from build123d import *

# Parameters (mm, degrees)
SKETCH_1_R          = 13.5
SKETCH_1_R_2        = 10
EXTRUDE_1_DEPTH     = 4
SKETCH_2_R          = 12.5
SKETCH_2_R_2        = 12.2
SKETCH_2_R_3        = 11.3
SKETCH_2_R_4        = 11
CUT_EXTRUDE_1_DEPTH = 0.3


with BuildPart() as part:
    # 草图1 → 凸台-拉伸1 (new body)
    with BuildSketch(Plane(origin=(0, 0, 0), x_dir=(1, 0, 0), z_dir=(0, 1, 0))):
        with Locations(Location((0, 0, 0), (0, 0, 270))):
            Circle(SKETCH_1_R)
        with Locations(Location((0, 0, 0), (0, 0, 270))):
            Circle(SKETCH_1_R_2, mode=Mode.SUBTRACT)
    extrude(amount=EXTRUDE_1_DEPTH)

    # 草图2 → 切除-拉伸1 (cut)
    # profile 1 of 2: a face of its own
    with BuildSketch(Plane(origin=(0, 4, 0), x_dir=(1, 0, 0), z_dir=(0, 1, 0))):
        with Locations(Location((0, 0, 0), (0, 0, 270))):
            Circle(SKETCH_2_R)
        with Locations(Location((0, 0, 0), (0, 0, 270))):
            Circle(SKETCH_2_R_2, mode=Mode.SUBTRACT)
    # profile 2 of 2: a face of its own
    with BuildSketch(Plane(origin=(0, 4, 0), x_dir=(1, 0, 0), z_dir=(0, 1, 0))):
        with Locations(Location((0, 0, 0), (0, 0, 270))):
            Circle(SKETCH_2_R_3)
        with Locations(Location((0, 0, 0), (0, 0, 270))):
            Circle(SKETCH_2_R_4, mode=Mode.SUBTRACT)
    cut_extrude_1 = extrude(amount=-CUT_EXTRUDE_1_DEPTH, mode=Mode.SUBTRACT)

    # 镜向1: 切除-拉伸1 across plane
    add(cut_extrude_1.mirror(Plane.ZX.offset(2)), mode=Mode.SUBTRACT)


solid = part.part
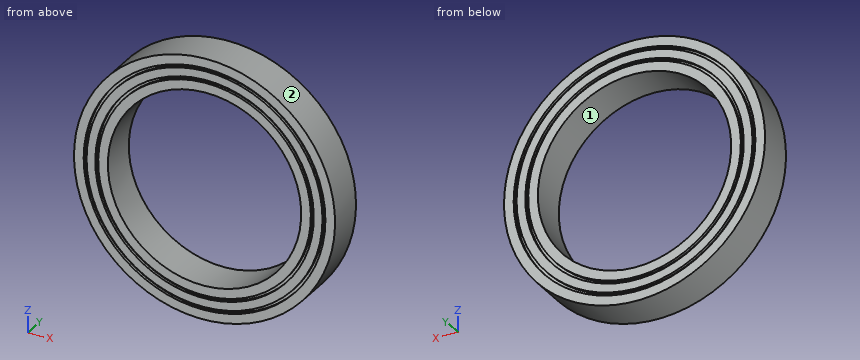
CAD build for the part. Positions are in the model's coordinates, mm. Face numbers are marked on the shaded views. Coordinates: 2 decimals unless noted, no trailing zeros. Loops run counter-clockwise (first coordinate to the right, second up) from the corner with the lowest first, then second, coordinate; pieces in that order, holes last. Notation, with made-up numbers: (-6, 36) -> (27, 36) arc R30 cw to (27, 74) -> close; hole circle Ø10 at (75.25, 37). An arc over 180 degrees is marked (long way). One line per item, written item: value.
1. Drill centre lines: line 1 (X direction, y = 3.9, z = 0); line 2 (Z direction, x = 7.75, y = 2.2). Where is each one in solid material? Low to high. Write a range as [from, to].
Answers:
line 1: x = [-13.5, -12.5], [-12.2, -11.3], [-11, -10], [10, 11], [11.3, 12.2], [12.5, 13.5]
line 2: z = [-11.05, -6.32], [6.32, 11.05]
2. Slice it at A-A on y = 2.4. Write the cut outline in (x, z).
Answers:
outline: circle Ø27 at (0, 0); hole circle Ø20 at (0, 0)
3. Pull direction X, two halves, no side cores. Call the marked faces 1 and 2: pulls with the +X half, pulls with the -X half, needs draft (parallel to the pull), parting line crosses it, or undercut.
Answers:
face 1: undercut
face 2: parting line crosses it
